Design review of the part built by this model. Coordinates are the model's own, in mm. Coordinates: 2 decimals unless noted, no trailing zeros. Order: outer loops, then holes, each group sorted by start corner. A loop starts at its lowest first (then second) coordinate and runs counter-clockwise, first axis right, second up. Notation, with made-up numbers: M -11,19.5 L 4,19.5 A15 cw 4,40.5 Z; hole C 74.5,-27 d1. An arc over 180 degrees is marked long. Answer in a Markdown table with one row per item.
from build123d import *

# Parameters (mm, degrees)
SKETCH1_W             = 1285
SKETCH1_H             = 100
BOSS_EXTRUDE1_DEPTH   = 10
CUT_EXTRUDE1_REACH    = 652.312
SKETCH_PATTERN1_DEPTH = 10


# Read off the part's stored shape, not the designer's step: Sketch-Pattern1
with BuildPart() as part:
    # Sketch1 → Boss-Extrude1 (new body)
    with BuildSketch(Plane.XY):
        with Locations((0, 50)):
            Rectangle(SKETCH1_W, SKETCH1_H)
    extrude(amount=BOSS_EXTRUDE1_DEPTH)

    # Sketch2 → Cut-Extrude1 (cut, up to next)
    with BuildSketch(Plane.XY.offset(10), mode=Mode.PRIVATE) as cut_extrude1_sk1:
        Polygon((-82.5, 125), (-27.5, 70), (27.5, 70), (82.5, 125), align=None)
    cut_extrude1_tool1 = extrude(cut_extrude1_sk1.sketch, amount=-CUT_EXTRUDE1_REACH, mode=Mode.PRIVATE) & part.part
    add(cut_extrude1_tool1.solids().sort_by_distance((0, 102.083333, 10))[0], mode=Mode.SUBTRACT)

    # Sketch-Pattern1 outline → Sketch-Pattern1 (cut)
    with BuildSketch(Plane.XY):
        Polygon((-559.5, 60), (-504.5, 60), (-464.5, 100), (-599.5, 100), align=None)
        Polygon((-203.5, 100), (-328.5, 100), (-293.5, 65), (-238.5, 65), align=None)
    sketch_pattern1 = extrude(amount=SKETCH_PATTERN1_DEPTH, mode=Mode.SUBTRACT)

    # Mirror1: Sketch-Pattern1 across plane
    add(sketch_pattern1.mirror(Plane(origin=(0, 0, 0), x_dir=(0, 0, 1), z_dir=(1, 0, 0))), mode=Mode.SUBTRACT)


solid = part.part
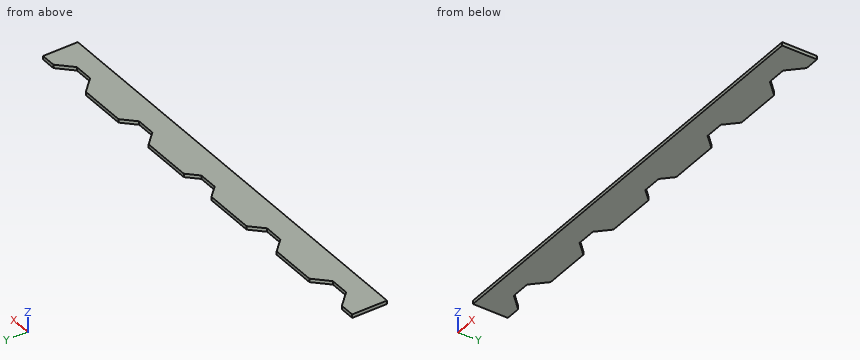
(1) Add section C-C, the plane x = -2. Give the boundary of the cut face in (y, z), and give its area (3 significant figures).
Return value:
| item | result |
|---|---|
| outline | M 0,0 L 70,0 L 70,10 L 0,10 Z |
| area | 700 mm2 |
(2) Insertion check: pin 1 Ø1 at (x, z) = (309.5, 7) entering from +Y; pin 2 Ø3 at (x, z) = (-3, 5.5) entering from +Y; pin 3 Ø5 at (x, z) = (28.5, 3.5) entering from +Y; pin 4 Ø8 at (x, y) = (471, 84) entering from -Z. Each pin has a flat end and moves straight along its axis. Give the tip position at first contact, or say it passes through.
Return value:
| item | result |
|---|---|
| pin 1 | stops at y = 81.5 |
| pin 2 | stops at y = 70 |
| pin 3 | stops at y = 73.5 |
| pin 4 | stops at z = 0 |
(3) For line 1 along X through (y, z) = (72.5, 0.75); line 2 along X through (y, z) = (89, 9); line 3 along X through (y, z) = (67, 3.5), list the stretches that pass through material, from the lowest coordinate up. Write a range as from..to.
Return value:
| item | result |
|---|---|
| line 1 | x = -642.5..-572, -492..-301, -231..-30, 30..231, 301..492, 572..642.5 |
| line 2 | x = -642.5..-588.5, -475.5..-317.5, -214.5..-46.5, 46.5..214.5, 317.5..475.5, 588.5..642.5 |
| line 3 | x = -642.5..-566.5, -497.5..-295.5, -236.5..236.5, 295.5..497.5, 566.5..642.5 |
(4) Add section A-A, the plane z = 6.25. Give the boundary of the cut face in (x, y), and give its area (3 significant figures).
Return value:
| item | result |
|---|---|
| outline | M -642.5,0 L 642.5,0 L 642.5,100 L 599.5,100 L 559.5,60 L 504.5,60 L 464.5,100 L 328.5,100 L 293.5,65 L 238.5,65 L 203.5,100 L 57.5,100 L 27.5,70 L -27.5,70 L -57.5,100 L -203.5,100 L -238.5,65 L -293.5,65 L -328.5,100 L -464.5,100 L -504.5,60 L -559.5,60 L -599.5,100 L -642.5,100 Z |
| area | 112,000 mm2 |
(5) Add section B-B, the plane x = -492.5. Give the boundary of the cut face in (y, z).
Return value:
| item | result |
|---|---|
| outline | M 0,0 L 72,0 L 72,10 L 0,10 Z |
